Source: three-view drawing plus pictorial views. Frame: mm from the lowest corner of the part. A direction names the side the tool comes from. Round coordinates to 2 decimals unless told otherwise and drop trailing zeros. Loops run counter-clockwise (first coordinate to the right, second up) from the corner with the lowest first, then second, coordinate; pieces in that order, holes last. Notation, with made-up numbers: M 25,59.25 L 35,59.25 A15 cw 35,83.25 Z; hole C 0,-29.75 d4. An arc over 180 degrees is marked long. Answer as a JSON object with one key per item and string values.
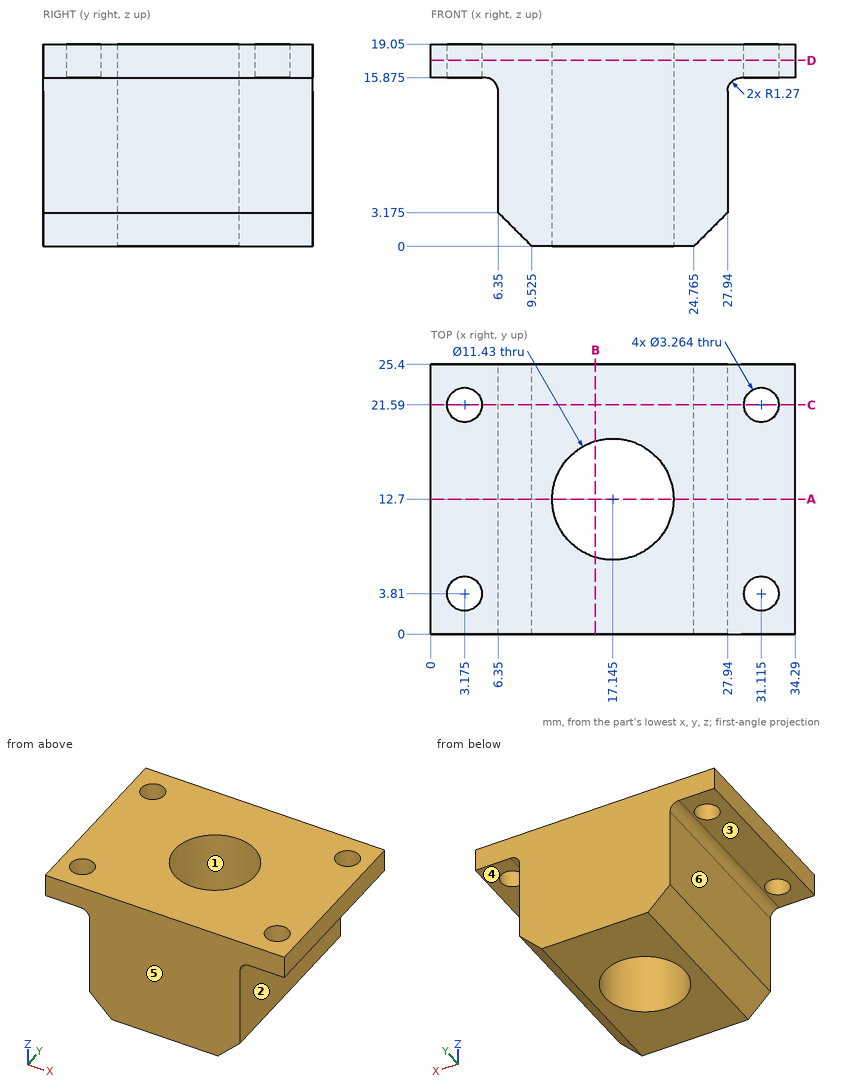
1) Set-up query: the marked faces 4, 5 and 6. Return all of +Z, -Z, +X, -X, +Y, -Y with unobstructed straight access to the full face (end or side cutting, diameter ignored); none if empty.
Geometry results:
{"face 4": "-Z, +X, +Y, -Y", "face 5": "+Z, -Z, +X, -X, -Y", "face 6": "-Z, -X, +Y, -Y"}
2) Pull-direction query (X, two-part tool) for the marked faces 1, 2 and 3; classes: +X half, -X half, draft (parallel to the pull), parting line (faces both ways), or undercut.
Geometry results:
{"face 1": "undercut", "face 2": "+X half", "face 3": "draft"}
3) First-contact query: pin 1 (4 mm diameter, centred on x = 3.175, y = 21.59, fed in from -Z); pin 2 (6 mm diameter, centred on x = 4, y = 5.5, fed in from -Z) (3 decimals); pin 3 (12 mm diameter, centred on x = 27.5, y = 19.5, fed in from -Z); pin 4 (1 mm diameter, centred on y = 5.5, z = 5.5, fed in from +X). Flat tips, straight axial feed; report the tip coordinate or a pass-through.
Geometry results:
{"pin 1": "z = 15.87", "pin 2": "z = 2.525", "pin 3": "z = 0", "pin 4": "x = 27.94"}
4) Line query: probe 1 along X at (y, z) = (12.75, 9.5); probe 2 along X at (y, z) = (1.5, 3.5); probe 3 along Y at (x, z) = (18, 15.5). Output: solid intervals per line, ascending.
Geometry results:
{"probe 1": "6.35 to 11.43, 22.86 to 27.94", "probe 2": "6.35 to 27.94", "probe 3": "0 to 7.05, 18.35 to 25.4"}
5) Cut plane B-B on x = 15.5. Return the cut outline in (y, z), and give its area (3 significant figures).
Geometry results:
{"outline": "M 0,0 L 7.23,0 L 7.23,19.05 L 0,19.05 Z; M 18.17,0 L 25.4,0 L 25.4,19.05 L 18.17,19.05 Z", "area": "275 mm2"}
6) Cut plane A-A on y = 12.7. Return the cut outline in (x, z) (3 decimals).
Geometry results:
{"outline": "M 0,15.875 L 5.08,15.875 A1.27 cw 6.35,14.605 L 6.35,3.175 L 9.525,0 L 11.43,0 L 11.43,19.05 L 0,19.05 Z; M 22.86,0 L 24.765,0 L 27.94,3.175 L 27.94,14.605 A1.27 cw 29.21,15.875 L 34.29,15.875 L 34.29,19.05 L 22.86,19.05 Z"}
7) Cut plane D-D on z = 17.5. Return the cut outline in (x, y) (3 decimals).
Geometry results:
{"outline": "M 0,0 L 34.29,0 L 34.29,25.4 L 0,25.4 Z; hole C 3.175,3.81 d3.264; hole C 3.175,21.59 d3.264; hole C 17.145,12.7 d11.43; hole C 31.115,3.81 d3.264; hole C 31.115,21.59 d3.264"}
8) Cut plane C-C on y = 21.59. Return the cut outline in (x, z) (3 decimals), and give its area (4 significant figures).
Geometry results:
{"outline": "M 0,15.875 L 1.543,15.875 L 1.543,19.05 L 0,19.05 Z; M 4.807,15.875 L 5.08,15.875 A1.27 cw 6.35,14.605 L 6.35,3.175 L 9.525,0 L 24.765,0 L 27.94,3.175 L 27.94,14.605 A1.27 cw 29.21,15.875 L 29.483,15.875 L 29.483,19.05 L 4.807,19.05 Z; M 32.747,15.875 L 34.29,15.875 L 34.29,19.05 L 32.747,19.05 Z", "area": "421.5 mm2"}
